Design review of the part built by this model. Coordinates are the model's own, in mm. Give positions to 0.01 mm unless a question says otherwise; leave off trailing zeros. Write each loop counter-clockwise with the first axis right and the second up, starting at its lowest first coordinate (ties: lowest second). Pieces come first, ordered by that corner, then holes. Notation, with made-up numbers: (-9.5, 30.5) - (29.5, 30.5) arc R21 cw to (29.5, 51.5) - close; hole circle Ø4 at (-12.5, 35). An arc over 180 degrees is marked (long way). Use a Markdown table: item, result. Add a question column.
```python
from build123d import *

# Parameters (mm, degrees)
SKETCH1_R           = 75
BOSS_EXTRUDE1_DEPTH = 400
FILLET1_R           = 10
FILLET2_R           = 10


with BuildPart() as part:
    # Sketch1 → Boss-Extrude1 (new body)
    with BuildSketch(Plane(origin=(0, 0, 0), x_dir=(1, 0, 0), z_dir=(0, 1, 0))):
        with Locations(Location((0, 0, 0), (0, 0, 90))):
            Circle(SKETCH1_R)
    extrude(amount=BOSS_EXTRUDE1_DEPTH)

    # Fillet1
    fillet1_edges = [part.edges().sort_by_distance(p)[0] for p in [
        (0, 400, 75),
    ]]
    fillet(fillet1_edges, radius=FILLET1_R)

    # Fillet2
    fillet2_edges = [part.edges().sort_by_distance(p)[0] for p in [
        (0, 0, 75),
    ]]
    fillet(fillet2_edges, radius=FILLET2_R)


solid = part.part
```
(1) For line 1 along Y through (x, z) = (59, 30); line 2 along X through (y, z) = (70.5, 30); line 3 along Z through (x, y) = (-29, 286.5), list the stretches that pass through material, from the lowest coordinate up.
(2) Insertion check: pin 1 (1 mm diameter, centred on y = 210, z = 44.5, fed in from -X); pin 2 (6 mm diameter, centred on x = 46, z = -56, fed in from -Y) (3 decimals); pin 3 (8 mm diameter, centred on x = 42, y = 79, fed in from -Z). Each pin has a flat end and moves straight along its axis. Give the tip position at first contact, or say it passes through.
(3) Add section A-A (y = 227.5). State the section outline as (x, z) points, and give its area (3 significant figures).
Answers follow:
| question | item | result |
|---|---|---|
| 1 | line 1 | 0.07 to 399.93 |
| 1 | line 2 | -68.74 to 68.74 |
| 1 | line 3 | -69.17 to 69.17 |
| 2 | pin 1 | x = -60.74 |
| 2 | pin 2 | y = 1.055 |
| 2 | pin 3 | z = -64.66 |
| 3 | outline | circle Ø150 at (0, 0) |
| 3 | area | 17,700 mm^2 |
